The model under review builds one solid part; all positions refer to its coordinate system, in mm. Face numbers are marked on the shaded views. A direction names the side the tool comes from. Round coordinates to 2 decimals unless told otherwise and drop trailing zeros. Write each loop counter-clockwise with the first axis right and the second up, starting at its lowest first coordinate (ties: lowest second). Pieces come first, ordered by that corner, then holes. Notation, with made-up numbers: (-29.5, 18) -> (-25.5, 18) arc R8 ccw to (-25.5, 24) -> close; hole circle Ø4 at (0, 69). An arc over 180 degrees is marked (long way). Use CSV: the item, a comma, the result in double quotes. Start each with the question number.
1) Take a section at B-B, the plane z = 0. Give the boundary of the cut face in (x, y), then the cut area to 3 significant figures.
2) Take a section at A-A, the plane x = 0. Give the boundary of the cut face in (y, z), then the cut area to 3 significant figures.
3) Take a section at D-D, the plane x = 6. Give the boundary of the cut face in (y, z).
4) For pin 1 Ø1 at (x, z) = (11, 7) entering from +Y; pin 2 Ø12 at (x, y) = (1.5, 28.5) entering from +Z; pin 3 Ø1 at (x, z) = (4.5, -16) entering from -Y, all flat-tipped, find the tip position at first contact; note any pin that passes through.
5) Mouldability with a two-part tool opening along Y and no side actions: class the marked faces 3, 4 and 5 as released by +Y, released by -Y, zero draft, split by the parting line, or undercut.
6) Wall thickness on probe 1 along X at (y, z) = (2.4, 0); probe 2 along Z at (x, y) = (-0.5, 21); probe 3 along Y at (x, z) = (-9, 11.5): over which ranges is each line inside the solid? List them lowest first. Write a range as [from, to].
7) Take a section at C-C, the plane y = 38. Give the boundary of the cut face in (x, z).
8) Machinability: for the marked faces 1 and 2, which of the approach directions +Z, -Z, +X, -X, +Y, -Y give a long, thin tool a straight path to every point of the face, cutting with its end or side? Answer none if there is none.
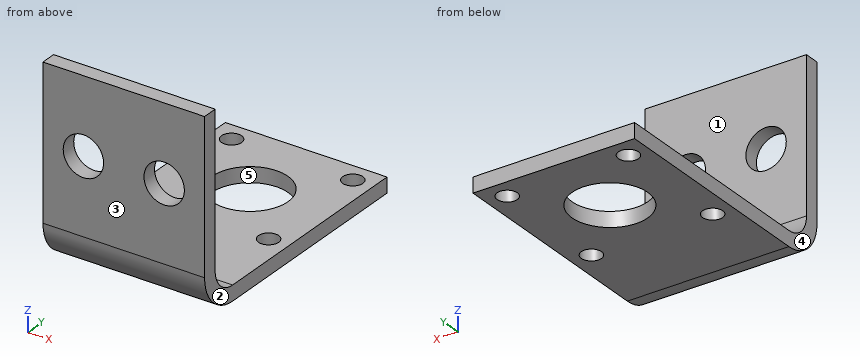
from build123d import *

# Parameters (mm, degrees)
SKETCH5_W          = 32
SKETCH5_H          = 30
BASE_FLANGE1_DEPTH = 3
EDGE_FLANGE1_DEPTH = 32
SKETCH13_R         = 4
CUT_EXTRUDE1_DEPTH = 10
SKETCH14_R         = 7.5
SKETCH14_R_2       = 2
CUT_EXTRUDE2_DEPTH = 10


# Sheet-metal steps are written as plain solids
with BuildPart() as part:
    # Sketch5 → Base-Flange1 (new body)
    with BuildSketch(Plane(origin=(0, 0, 0), x_dir=(1, 0, 0), z_dir=(0, 1, 0))):
        Rectangle(SKETCH5_W, SKETCH5_H)
    extrude(amount=BASE_FLANGE1_DEPTH)

    # Edge-Flange1 section (across the edge) → Edge-Flange1 (add)
    with BuildSketch(Plane(origin=(16, 3, -20), x_dir=(0, 0, 1), z_dir=(-1, 0, 0))):
        with BuildLine():
            Line((-3, 5), (-3, 49))
            Line((-3, 49), (0, 49))
            Line((0, 49), (0, 5))
            ThreePointArc((0, 5), (1.464466094, 1.464466094), (5, 0))
            Line((5, 0), (5, -3))
            ThreePointArc((5, -3), (-0.656854249, -0.656854249), (-3, 5))
        make_face()
    extrude(amount=EDGE_FLANGE1_DEPTH)

    # Sketch13 → Cut-Extrude1 (cut)
    with BuildSketch(Plane(origin=(0, 3, 0), x_dir=(1, 0, 0), z_dir=(0, 1, 0))):
        with Locations(Location((-8, 0, 0), (0, 0, 270))):
            Circle(SKETCH13_R)
        with Locations(Location((8, 0, 0), (0, 0, 270))):
            Circle(SKETCH13_R)
    extrude(amount=-CUT_EXTRUDE1_DEPTH, mode=Mode.SUBTRACT)

    # Sketch14 → Cut-Extrude2 (cut)
    with BuildSketch(Plane.XY.offset(-20)):
        with Locations((0, 36)):
            Circle(SKETCH14_R)
        with Locations((-12, 48)):
            Circle(SKETCH14_R_2)
        with Locations(Location((12, 48, 0), (0, 0, 270))):
            Circle(SKETCH14_R_2)
        with Locations((12, 24)):
            Circle(SKETCH14_R_2)
        with Locations(Location((-12, 24, 0), (0, 0, 270))):
            Circle(SKETCH14_R_2)
    extrude(amount=-CUT_EXTRUDE2_DEPTH, mode=Mode.SUBTRACT)


solid = part.part
Values found:
1,outline,"(-16, 0) -> (-12, 0) -> (-12, 3) -> (-16, 3) -> close; (-4, 0) -> (4, 0) -> (4, 3) -> (-4, 3) -> close; (12, 0) -> (16, 0) -> (16, 3) -> (12, 3) -> close"
1,area,"48.0 mm²"
2,outline,"(0, -15) arc R8 ccw to (8, -23) -> (28.5, -23) -> (28.5, -20) -> (8, -20) arc R5 cw to (3, -15) -> (3, 15) -> (0, 15) -> close; (43.5, -23) -> (52, -23) -> (52, -20) -> (43.5, -20) -> close"
2,area,"208 mm²"
3,outline,"(0, -15) arc R8 ccw to (8, -23) -> (31.5, -23) -> (31.5, -20) -> (8, -20) arc R5 cw to (3, -15) -> (3, -3.46) -> (0, -3.46) -> close; (0, 3.46) -> (3, 3.46) -> (3, 15) -> (0, 15) -> close; (40.5, -23) -> (52, -23) -> (52, -20) -> (40.5, -20) -> close"
4,pin 1,"y = 3"
4,pin 2,"z = -20"
4,pin 3,"y = 0.02"
5,face 3,"released by -Y"
5,face 4,"zero draft"
5,face 5,"undercut"
6,probe 1,"[-16, -12], [-4, 4], [12, 16]"
6,probe 2,"[-23, -20]"
6,probe 3,"[0, 3]"
7,outline,"(-16, -23) -> (-7.23, -23) -> (-7.23, -20) -> (-16, -20) -> close; (7.23, -23) -> (16, -23) -> (16, -20) -> (7.23, -20) -> close"
8,face 1,"+Z, +X, -X, +Y"
8,face 2,"+Z, -Z, +X, +Y, -Y"
